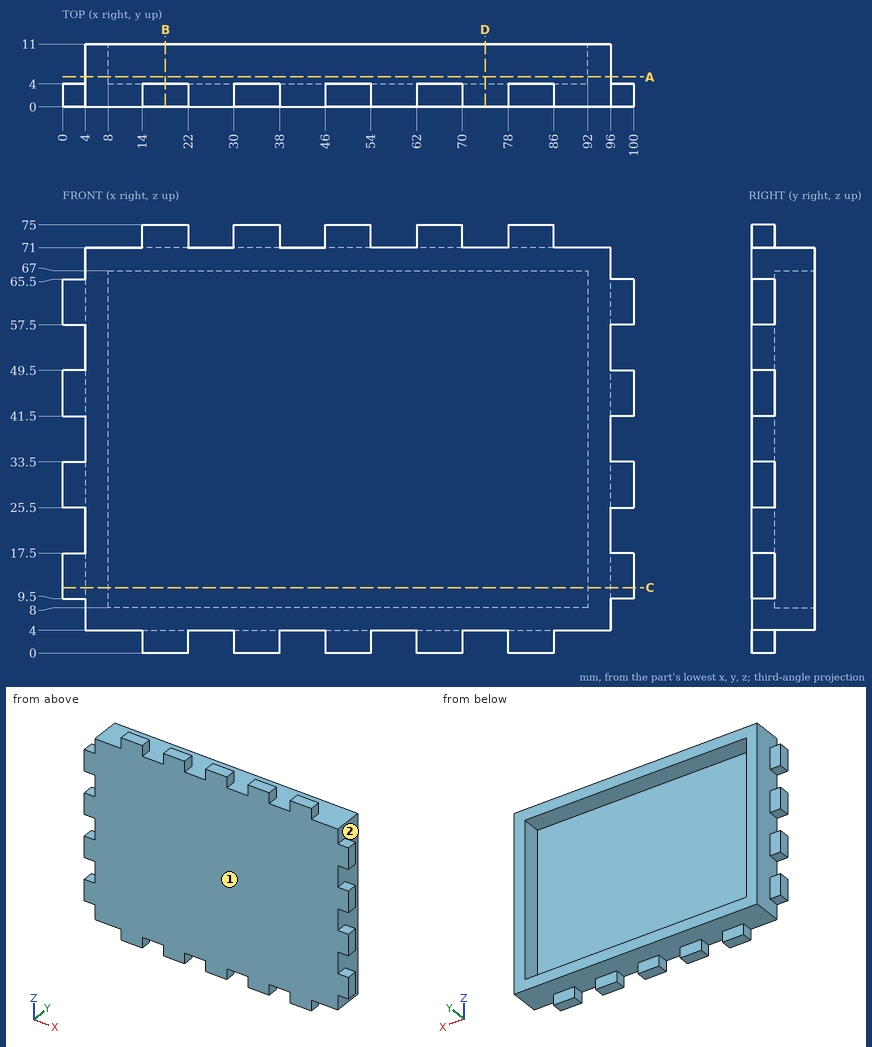
Here's the drawing with two shaded views (mm, measured from the low corner). I have some questions. Coordinates: 2 decimals unless noted, no trailing zeros. Order: outer loops, then holes, each group sorted by start corner. A loop starts at its lowest first (then second) coordinate and runs counter-clockwise, first axis right, second up. Notation, with made-up numbers: (-29.5, 42) - (7.5, 42) arc R19 cw to (7.5, 63) - close; hole circle Ø1 at (79.5, 81). An arc over 180 degrees is marked (long way). Answer in a Markdown table with one row per item.
1. If we mould it in two halves opening along Z, with no side actions, what happens to the marked faces 1 and 2? For each: pulls with the +Z half, pulls with the -Z half, needs draft (parallel to the pull), parting line crosses it, or undercut.
Reply:
| item | result |
|---|---|
| face 1 | needs draft |
| face 2 | undercut |
2. For pin 1 (1 mm diameter, centred on y = 6.5, z = 30, fed in from -X); pin 2 (8 mm diameter, centred on x = 86.5, z = 24.5, fed in from +Y); pin 3 (4.5 mm diameter, centred on y = 1, z = 72, fed in from +X), each with a flat end and sliding along its axis, tell me the tip position at first contact or that it passes through.
Reply:
| item | result |
|---|---|
| pin 1 | stops at x = 4 |
| pin 2 | stops at y = 4 |
| pin 3 | stops at x = 96 |
3. If I drill on line 1 along Z through (x, y) = (78, 4.75); line 2 along X through (y, z) = (8.5, 30.5); line 3 along Y through (x, z) = (35.5, 21), over which ranges is the centre line in solid material (lowest first)?
Reply:
| item | result |
|---|---|
| line 1 | z = 4 to 8, 67 to 71 |
| line 2 | x = 4 to 8, 92 to 96 |
| line 3 | y = 0 to 4 |
4. Suppose I cut it at C-C (z = 11.5). Please give me the cut outline in (x, y), and give its area (3 significant figures).
Reply:
| item | result |
|---|---|
| outline | (0, 0) - (100, 0) - (100, 4) - (96, 4) - (96, 11) - (92, 11) - (92, 4) - (8, 4) - (8, 11) - (4, 11) - (4, 4) - (0, 4) - close |
| area | 456 mm^2 |
5. Suppose I cut it at D-D (x = 74). Please give me the cut outline in (y, z).
Reply:
| item | result |
|---|---|
| outline | (0, 4) - (11, 4) - (11, 8) - (4, 8) - (4, 67) - (11, 67) - (11, 71) - (0, 71) - close |
6. Suppose I cut it at B-B (x = 18). Please give me the cut outline in (y, z).
Reply:
| item | result |
|---|---|
| outline | (0, 0) - (4, 0) - (4, 4) - (11, 4) - (11, 8) - (4, 8) - (4, 67) - (11, 67) - (11, 71) - (4, 71) - (4, 75) - (0, 75) - close |
7. Suppose I cut it at A-A (y = 5.25). Please give me the cut outline in (x, z), and give its area (3 significant figures).
Reply:
| item | result |
|---|---|
| outline | (4, 4) - (96, 4) - (96, 71) - (4, 71) - close; hole (8, 8) - (92, 8) - (92, 67) - (8, 67) - close |
| area | 1,210 mm^2 |
